The drawing under review shows one solid part. Ordinate dimensions are in mm from its lowest x, y, z. A direction names the side the tool comes from. Give positions to 0.01 mm unless a question says otherwise; leave off trailing zeros. Order: outer loops, then holes, each group sorted by start corner. A loop starts at its lowest first (then second) coordinate and runs counter-clockwise, first axis right, second up. Notation, with made-up numbers: (-38, 65) - (17, 65) arc R29 cw to (17, 94) - close; hole circle Ø5 at (41.25, 82). An arc over 180 degrees is marked (long way). Write item = value, one per line. Start each with the question number.
1. Machinability: for the marked faces 4 and 5, which of the approach directions +Z, -Z, +X, -X, +Y, -Y give a long, thin tool a straight path to every point of the face, cutting with its end or side? Answer none if there is none.
2. We need section D-D, the plane z = 0.75. Give the boundary of the cut face in (x, y).
3. We need section C-C, the plane x = 8.5. Give the boundary of the cut face in (y, z), and give its area (3 significant figures).
4. We need section A-A, the plane y = 11.5. Give the boundary of the cut face in (x, z).
5. Mouldability with a two-part tool opening along X and no side actions: class the marked faces 1, 2 and 3 as pulls with the +X half, pulls with the -X half, needs draft (parallel to the pull), parting line crosses it, or undercut.
6. Wall thickness on probe 1 along Y at (x, z) = (11.5, 1.4); probe 2 along Z at (x, y) = (9.5, 2.5); probe 3 along Y at (x, z) = (16, 2.75): over which ranges is each line inside the solid? List them lowest first.
7. For P1, Ø12.5, axis at x = 11.5, y = 11.5, coming from the +Z side; P2, Ø2, axis at y = 7, z = 4, coming from the -X side; P3, Ø1, axis at x = 13, z = 7.5, coming from the -Y side; P4, Ø3, axis at x = 11.5, y = 11.5, coming from the -Z side, all flat-tipped, find the tip position at first contact; note any pin that passes through.
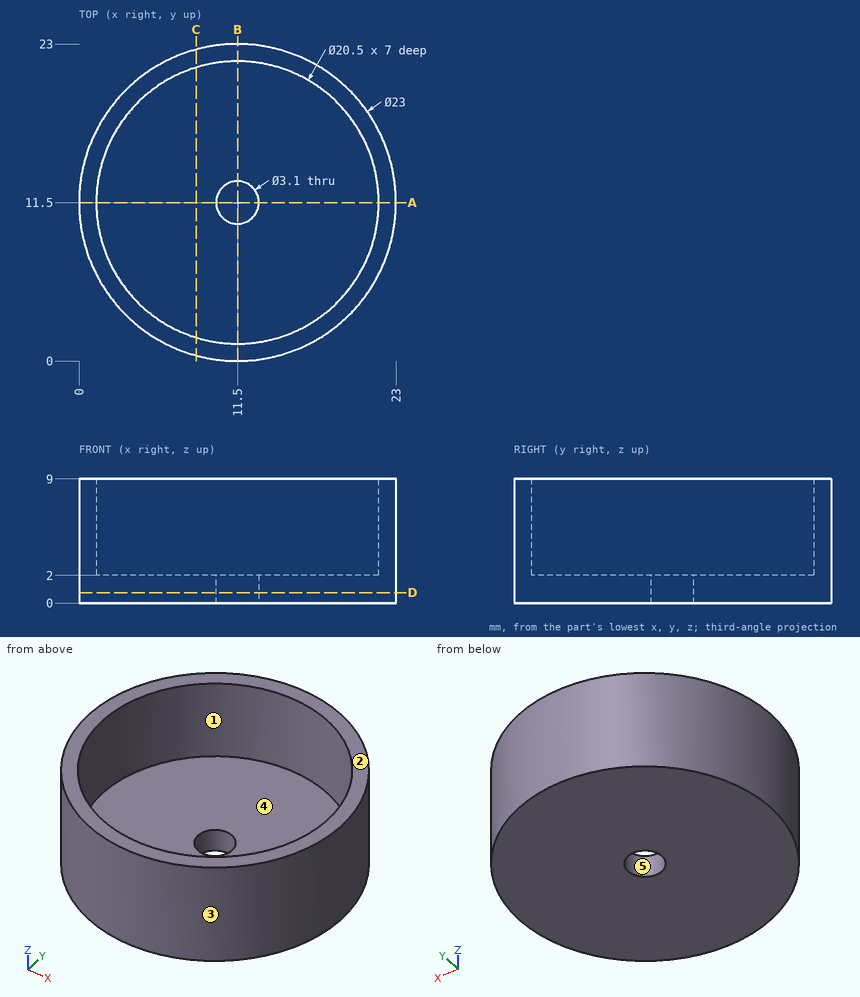
Model answer:
q1.face_4 = +Z
q1.face_5 = +Z, -Z
q2.outline = circle Ø23 at (11.5, 11.5); hole circle Ø3.1 at (11.5, 11.5)
q3.outline = (0.4, 0) - (22.6, 0) - (22.6, 9) - (21.3, 9) - (21.3, 2) - (1.7, 2) - (1.7, 9) - (0.4, 9) - close
q3.area = 62.6 mm2
q4.outline = (0, 0) - (9.95, 0) - (9.95, 2) - (1.25, 2) - (1.25, 9) - (0, 9) - close; (13.05, 0) - (23, 0) - (23, 9) - (21.75, 9) - (21.75, 2) - (13.05, 2) - close
q5.face_1 = undercut
q5.face_2 = needs draft
q5.face_3 = parting line crosses it
q6.probe_1 = 0 to 9.95, 13.05 to 23
q6.probe_2 = 0 to 2
q6.probe_3 = 0.92 to 2.29, 20.71 to 22.08
q7.P1 = 2
q7.P2 = 0.55
q7.P3 = 0.04
q7.P4 = through
